```python
from build123d import *

# Parameters (mm, degrees)
SKETCH1_R                = 29
BOSS_EXTRUDE1_DEPTH      = 53
SKETCH2_R                = 25
CUT_EXTRUDE1_DEPTH       = 68.014923711
CUT_EXTRUDE1_TAPER       = 5
EXTRUDE_START            = -5
SKETCH_1_R               = 39
SKETCH_1_R_2             = 29
EXTRUDE_1_DEPTH          = 5
EXTRUDE_START_2          = -10
SKETCH_2_R               = 39
SKETCH_2_R_2             = 29
EXTRUDE_2_DEPTH          = 10
CUT_EXTRUDE_1_REACH      = 108.705
CUT_EXTRUDE_1_END_RADIUS = 29
SKETCH_3_W               = 6.2
SKETCH_3_H               = 20.212278325
PATTERN_CIRCULAR_1_COUNT = 4


with BuildPart() as part:
    # Sketch1 → Boss-Extrude1 (new body)
    with BuildSketch(Plane.XY):
        Circle(SKETCH1_R)
    extrude(amount=-BOSS_EXTRUDE1_DEPTH)

    # Sketch2 → Cut-Extrude1 (cut, through all)
    with BuildSketch(Plane(origin=(0, 0, 0), x_dir=(-1, 0, 0), z_dir=(0, 0, -1))):
        Circle(SKETCH2_R)
    extrude(amount=CUT_EXTRUDE1_DEPTH, taper=CUT_EXTRUDE1_TAPER, mode=Mode.SUBTRACT)

    # Sketch3 → Cut-Revolve1 (revolve, cut)
    with BuildSketch(Plane(origin=(0, 0, 0), x_dir=(0, 0, -1), z_dir=(1, 0, 0)), mode=Mode.PRIVATE) as cut_revolve1_sk:
        with BuildLine():
            Line((41.5, 22), (41.5, 20.5))
            Line((41.5, 20.5), (38.5, 20.5))
            Line((38.5, 20.5), (38.5, 22))
            ThreePointArc((38.5, 22), (40, 23.5), (41.5, 22))
        make_face()
    revolve(cut_revolve1_sk.sketch.rotate(Axis((0, 0, -33.171853518), (0, 0, 1)), 90), axis=Axis((0, 0, -33.171853518), (0, 0, 1)), mode=Mode.SUBTRACT)

    # Sketch 1 → Extrude 1 (add)
    with BuildSketch(Plane(origin=(0, 0, -53), x_dir=(-1, 0, 0), z_dir=(0, 0, -1)).offset(EXTRUDE_START)):
        Circle(SKETCH_1_R)
        with Locations(Location((0, 0, 0), (0, 0, 180))):
            Circle(SKETCH_1_R_2, mode=Mode.SUBTRACT)
    extrude(amount=EXTRUDE_1_DEPTH)

    # Sketch 2 → Extrude 2 (add)
    with BuildSketch(Plane(origin=(0, 0, -38), x_dir=(-1, 0, 0), z_dir=(0, 0, -1)).offset(EXTRUDE_START_2)):
        Circle(SKETCH_2_R)
        with Locations(Location((0, 0, 0), (0, 0, 180))):
            Circle(SKETCH_2_R_2, mode=Mode.SUBTRACT)
    extrude(amount=EXTRUDE_2_DEPTH)

    # Cut-Extrude 1: up to this cylinder (the profile starts outside it)
    cut_extrude_1_end = Plane(origin=(0, 0, -32.476974), z_dir=(0, 0, 1)) * Cylinder(CUT_EXTRUDE_1_END_RADIUS, 276.41, mode=Mode.PRIVATE)
    # Sketch 3 → Cut-Extrude 1 (cut, up to the surface)
    with BuildSketch(Plane(origin=(0, 45, 0), x_dir=(1, 0, 0), z_dir=(0, 1, 0)), mode=Mode.PRIVATE) as cut_extrude_1_sk1:
        with Locations((0, 32.47697446)):
            Rectangle(SKETCH_3_W, SKETCH_3_H)
    cut_extrude_1_tool1 = extrude(cut_extrude_1_sk1.sketch, amount=-CUT_EXTRUDE_1_REACH, mode=Mode.PRIVATE) - cut_extrude_1_end
    cut_extrude_1 = cut_extrude_1_tool1.solids().sort_by_distance((0, 45, -32.476974))[0]
    add(cut_extrude_1, mode=Mode.SUBTRACT)

    # Pattern Circular 1: Cut-Extrude 1 ×4 about axis
    pattern_circular_1_axis = Axis((0, 0, 0), (0, 0, 1))
    for i in range(1, PATTERN_CIRCULAR_1_COUNT):
        add(cut_extrude_1.rotate(pattern_circular_1_axis, i * 360 / PATTERN_CIRCULAR_1_COUNT), mode=Mode.SUBTRACT)


solid = part.part
```
Part model, mm, in its own coordinate system. A direction names the side the tool comes from. Round coordinates to 2 decimals unless told otherwise and drop trailing zeros. Write each loop counter-clockwise with the first axis right and the second up, starting at its lowest first coordinate (ties: lowest second). Pieces come first, ordered by that corner, then holes. Notation, with made-up numbers: M 86.25,56 L 119.25,56 A14 cw 119.25,74 Z; hole C 57,77 d2. An arc over 180 degrees is marked long. Answer as CSV lines item,"result". Start each with the question number.
1) Band-saw the part on D-D (y = 27.5). List the corners of the cut face in (x, z).
2) Drill centre lines: L1, parallel to Z at x = 23, y = 30; L2, parallel to X at y = 5, z = -23.5; L3, parallel to Z at x = -21.5, y = 1. Where is each one in solid material? Low to high.
3) Band-saw the part on C-C (z = -35). List the corners of the cut face in (x, y).
4) Drop flat-ended pins along their axis: pin 1 (11 mm diameter, centred on y = -35.5, z = -35.5, fed in from -X); pin 2 (6 mm diameter, centred on x = 17.5, z = -34, fed in from +Y); pin 3 (11 mm diameter, centred on x = 36, z = -33, fed in from +Y); pin 4 (4 mm diameter, centred on x = -5.5, y = -15.5, fed in from +Z). Give the stop position or say it passes through.
5) Which spindle directions (+Z, -Z, +X, -X, +Y, -Y) get a long thin tool onto all of the face, cutting with end or side? Do faces 1 (the face through (21, 21, -38)), 2 (the face through (-21, 21, -38)), 3 (the face through (-20, 21, -24)), 4 (the face through (-3.1, -34, -33)), 5 (the face through (-21, 21, -28)). Say none if no direction does.
6) Band-saw the part on B-B (x = 0). List the corners of the cut face in (y, z), then the cut area to 3 significant figures.
7) Band-saw the part on A-A (y = -33). List the corners of the cut face in (x, z).
8) Mould opens along Y. For faces 6 (the face through (3.1, 34, -33)), 7 (the face through (27.3, 27.85, -32.93)), 8 (the face through (16.2, 14.6, -38.5)), 9 (the face through (18, -12, -41.5)) say: +Y half, -Y half, draft (parallel to the pull), parting line (faces both ways), or undercut.
Worked out:
1,outline,"M -27.65,-53 L 27.65,-53 L 27.65,-48 L 9.21,-48 L 9.21,-38 L 27.65,-38 L 27.65,-28 L 9.21,-28 L 9.21,0 L -9.21,0 L -9.21,-28 L -27.65,-28 L -27.65,-38 L -9.21,-38 L -9.21,-48 L -27.65,-48 Z"
2,L1,"-53 to -48, -38 to -28"
2,L2,"-28.57 to -22.39, 22.39 to 28.57"
2,L3,"-53 to -41.5"
3,outline,"M -38.88,-3.1 A39 ccw -3.1,-38.88 L -3.1,-28.83 A29 ccw 3.1,-28.83 L 3.1,-38.88 A39 ccw 38.88,-3.1 L 28.83,-3.1 A29 ccw 28.83,3.1 L 38.88,3.1 A39 ccw 3.1,38.88 L 3.1,28.83 A29 ccw -3.1,28.83 L -3.1,38.88 A39 ccw -38.88,3.1 L -28.83,3.1 A29 ccw -28.83,-3.1 Z; hole C 0,0 d43.88"
4,pin 1,"x = -24.92"
4,pin 2,"y = 36.2"
4,pin 3,"y = 24.31"
4,pin 4,"through"
5,face 1,"+X, +Y"
5,face 2,"-X, +Y"
5,face 3,"none"
5,face 4,"+Z, -Y"
5,face 5,"+Z, -X, +Y"
6,outline,"M -39,-53 L -20.36,-53 L -21.37,-41.5 L -22,-41.5 A1.5 cw -22,-38.5 L -21.63,-38.5 L -25,0 L -29,0 L -29,-48 L -39,-48 Z; M 20.36,-53 L 39,-53 L 39,-48 L 29,-48 L 29,0 L 25,0 L 21.63,-38.5 L 22,-38.5 A1.5 cw 22,-41.5 L 21.37,-41.5 Z"
6,area,"760 mm²"
7,outline,"M -20.78,-53 L 20.78,-53 L 20.78,-48 L -20.78,-48 Z; M -20.78,-38 L -3.1,-38 L -3.1,-28 L -20.78,-28 Z; M 3.1,-38 L 20.78,-38 L 20.78,-28 L 3.1,-28 Z"
8,face 6,"draft"
8,face 7,"+Y half"
8,face 8,"undercut"
8,face 9,"undercut"
